```python
from build123d import *

# Parameters (mm, degrees)
F0_W     = 279.4
F0_H     = 177.8
F1_DEPTH = 25.4
F2_W     = 279.4
F2_H     = 12.7
F3_DEPTH = 12.7
F4_W     = 279.4
F4_H     = 12.7
F5_DEPTH = 12.7
F6_W     = 12.7
F6_H     = 88.9
F7_DEPTH = 12.7
F8_W     = 12.7
F8_H     = 88.9
F9_DEPTH = 12.7


with BuildPart() as f1:
    # F0 (on Right) → F1 (new body)
    with BuildSketch(Plane.YZ):
        with Locations((-139.7, 88.9)):
            Rectangle(F0_W, F0_H)
    extrude(amount=F1_DEPTH)

    # F2 (on face) → F3 (cut)
    with BuildSketch(Plane(origin=(0, 0, 0), x_dir=(0, -1, 0), z_dir=(-1, 0, 0))):
        with Locations((139.7, 12.7)):
            Rectangle(F2_W, F2_H)
    extrude(amount=-F3_DEPTH, mode=Mode.SUBTRACT)

    # F4 (on face) → F5 (cut)
    with BuildSketch(Plane(origin=(0, 0, 0), x_dir=(0, -1, 0), z_dir=(-1, 0, 0))):
        with Locations((139.7, 165.1)):
            Rectangle(F4_W, F4_H)
    extrude(amount=-F5_DEPTH, mode=Mode.SUBTRACT)

    # F6 (on face) → F7 (join)
    with BuildSketch(Plane(origin=(0, 0, 0), x_dir=(-1, 0, 0), z_dir=(0, 1, 0))):
        with Locations((-12.7, 88.9)):
            Rectangle(F6_W, F6_H)
    extrude(amount=F7_DEPTH)

    # F8 (on face) → F9 (join)
    with BuildSketch(Plane.XZ.offset(279.4)):
        with Locations((12.7, 88.9)):
            Rectangle(F8_W, F8_H)
    extrude(amount=F9_DEPTH)


solid = f1.part
```
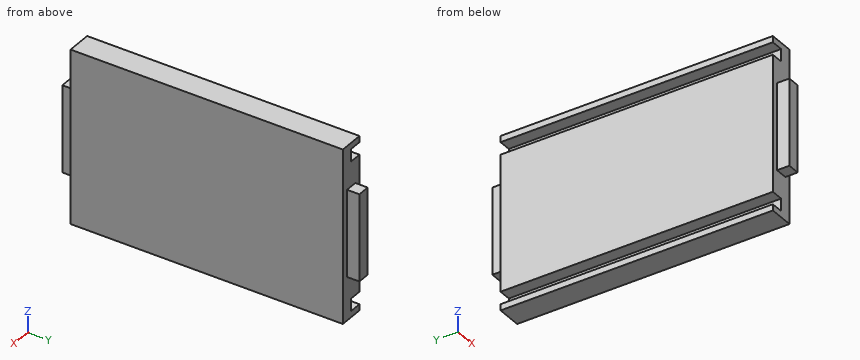
Verification items for the finished model (mm, model axes). Coordinates: 2 decimals unless noted, no trailing zeros. Order: outer loops, then holes, each group sorted by start corner. A loop starts at its lowest first (then second) coordinate and runs counter-clockwise, first axis right, second up. Notation, with made-up numbers: (-3, -28) -> (29, -28) arc R32 ccw to (29, 4) -> close; hole circle Ø11 at (-0.75, 61). An arc over 180 degrees is marked (long way). Put each result on its own line as item: value. Start each with the question number.
1) Cross-section at B-B (z = 127.5). Enter the section's corners in (x, y), plus the area to 3 significant figures.
2) Material ranges on L1, parallel to Z at x = 12, y = -138; L2, parallel to Y at x = 3.25, z = 72.5; L3, parallel to X at y = -265.5, z = 163.5, recorded low to high.
3) Cross-section at C-C (x = 22.5). Enter the section's corners in (y, z).
4) Go/stop test with flat-tipped pins: pin 1 (10 mm diameter, centred on y = -184.5, z = 164, fed in from -X); pin 2 (10 mm diameter, centred on y = 6.5, z = 90.5, fed in from -X); pin 3 (14 mm diameter, centred on y = 9.5, z = 105.5, fed in from +X). Record where each tip stops, or that it passes through.
5) Cross-section at D-D (z = 25). Enter the section's corners in (x, y), plus the area to 3 significant figures.
6) Cross-section at A-A (y = -214). Enter the section's corners in (x, z), plus the area to 3 significant figures.
Geometry check:
1. outline: (0, -279.4) -> (6.35, -279.4) -> (6.35, -292.1) -> (19.05, -292.1) -> (19.05, -279.4) -> (25.4, -279.4) -> (25.4, 0) -> (19.05, 0) -> (19.05, 12.7) -> (6.35, 12.7) -> (6.35, 0) -> (0, 0) -> close
1. area: 7,420 mm^2
2. L1: z = 0 to 6.35, 19.05 to 158.75, 171.45 to 177.8
2. L2: y = -279.4 to 0
2. L3: x = 12.7 to 25.4
3. outline: (-279.4, 0) -> (0, 0) -> (0, 177.8) -> (-279.4, 177.8) -> close
4. pin 1: stops at x = 12.7
4. pin 2: stops at x = 6.35
4. pin 3: stops at x = 19.05
5. outline: (0, -279.4) -> (25.4, -279.4) -> (25.4, 0) -> (0, 0) -> close
5. area: 7,100 mm^2
6. outline: (0, 0) -> (25.4, 0) -> (25.4, 177.8) -> (0, 177.8) -> (0, 171.45) -> (12.7, 171.45) -> (12.7, 158.75) -> (0, 158.75) -> (0, 19.05) -> (12.7, 19.05) -> (12.7, 6.35) -> (0, 6.35) -> close
6. area: 4,190 mm^2
